Autodesk Inventor part; units mm, degrees
ref_plane "YZ Plane" through (0, 0, 0) normal (1, 0, 0) x (0, 1, 0)
ref_plane "XZ Plane" through (0, 0, 0) normal (0, 1, 0) x (-1, 0, 0)
ref_plane "XY Plane" through (0, 0, 0) normal (0, 0, 1) x (1, 0, 0)
sketch "Sketch1" plane through (0, 0, 0) normal (1, 0, 0) x (0, 1, 0)
  line L0 (1.5875, 103.1875) -> (1.5875, 1.5875)
  line L1 (1.5875, 1.5875) -> (179.3875, 1.5875)
  line L2 (179.3875, 1.5875) -> (179.3875, 7.9375)
  line L3 (179.3875, 7.9375) -> (180.975, 7.9375)
  line L4 (180.975, 7.9375) -> (180.975, 0)
  line L5 (180.975, 0) -> (0, 0)
  line L6 (0, 0) -> (0, 103.1875)
  line L7 (0, 103.1875) -> (1.5875, 103.1875)
  dimension "d0" = 1.5875
  dimension "d1" = 1.5875
  dimension "d2" = 180.975
  dimension "d3" = 101.6
  dimension "d4" = 6.35
extrude "Extrusion1" add sketch "Sketch1" along normal blind 241.3
sketch "Sketch2" plane through (0, 0, 0) normal (0, 0, -1) x (-1, 0, 0)
  line L0 (-241.3, 180.975) -> (-241.3, 0)
  line L1 (0, 0) -> (-241.3, 0)
  line L2 (0, 0) -> (0, 180.975)
  line L3 (-241.3, 127) -> (-215.9, 127)
  line L4 (-215.9, 127) -> (-215.9, 76.2)
  line L5 (-215.9, 76.2) -> (-241.3, 76.2)
  line L6 (-241.3, 76.2) -> (-241.3, 127)
  line L7 (0, 127) -> (-25.4, 127)
  line L8 (-25.4, 127) -> (-25.4, 76.2)
  line L9 (-25.4, 76.2) -> (0, 76.2)
  line L10 (0, 76.2) -> (0, 127)
  dimension "d7" = 25.4
  dimension "d8" = 50.8
  dimension "d9" = 76.2
extrude "Extrusion2" cut sketch "Sketch2" against normal up to next
sketch "Sketch3" plane through (0, 1.5875, 1.5875) normal (0, 0, 1) x (1, 0, 0)
  line L0 (0, 125.4125) -> (25.4, 125.4125)
  line L1 (241.3, 74.6125) -> (215.9, 74.6125)
  line L2 (215.9, 125.4125) -> (214.3125, 125.4125)
  line L3 (214.3125, 125.4125) -> (214.3125, 74.6125)
  line L4 (214.3125, 74.6125) -> (215.9, 74.6125)
  line L5 (215.9, 74.6125) -> (215.9, 125.4125)
  line L6 (25.4, 74.6125) -> (26.9875, 74.6125)
  line L7 (26.9875, 74.6125) -> (26.9875, 125.4125)
  line L8 (26.9875, 125.4125) -> (25.4, 125.4125)
  line L9 (25.4, 125.4125) -> (25.4, 74.6125)
  point P0 (0, -1.5875)
  dimension "d12" = 1.5875
extrude "Extrusion3" add sketch "Sketch3" along normal blind 25.4
sketch "Sketch4" plane through (0, 179.3875, 1.5875) normal (0, 0, 1) x (1, 0, 0)
  line L0 (0, 0) -> (0, -52.3875)
  line L1 (241.3, -177.8) -> (241.3, -103.1875)
  circle A0 centre (228.6, -23.8125) radius 3.1877
  circle A1 centre (228.6, -125.4125) radius 3.1877
  circle A2 centre (12.7, -23.8125) radius 3.1877
  circle A3 centre (12.7, -125.4125) radius 3.1877
  line L2 (12.7, -23.8125) -> (228.6, -23.8125) construction
  line L3 (228.6, -23.8125) -> (228.6, -125.4125) construction
  line L4 (228.6, -125.4125) -> (12.7, -125.4125) construction
  line L5 (12.7, -125.4125) -> (12.7, -23.8125) construction
  line L6 (0, -179.3875) -> (241.3, -179.3875) construction
  line L7 (0, 1.5875) -> (241.3, 1.5875) construction
  dimension "d15" = 6.3754
  dimension "d16" = 12.7
  dimension "d18" = 25.4
  dimension "d19" = 101.6
  dimension "d20" = 12.7
extrude "Extrusion4" cut sketch "Sketch4" against normal through all
sketch "Sketch5" plane through (0, 0, 0) normal (0, -1, 0) x (1, 0, 0)
  line L0 (0, 103.1875) -> (31.75, 103.1875)
  line L1 (31.75, 103.1875) -> (31.75, 71.4375)
  line L2 (31.75, 71.4375) -> (0, 71.4375)
  line L3 (0, 71.4375) -> (0, 103.1875)
  line L4 (241.3, 103.1875) -> (209.55, 103.1875)
  line L5 (209.55, 103.1875) -> (209.55, 71.4375)
  line L6 (209.55, 71.4375) -> (241.3, 71.4375)
  line L7 (241.3, 71.4375) -> (241.3, 103.1875)
  dimension "d23" = 31.75
extrude "Extrusion5" cut sketch "Sketch5" against normal up to next
sketch "Sketch6" plane through (0, 1.5875, 1.5875) normal (0, 1, 0) x (1, 0, 0)
  line L0 (209.55, -101.6) -> (209.55, -69.85)
  line L1 (31.75, -69.85) -> (31.75, -101.6)
  line L2 (31.75, -101.6) -> (209.55, -101.6)
  circle A0 centre (76.2, -88.9) radius 3.175
  circle A1 centre (165.1, -88.9) radius 3.175
  line L3 (165.1, -88.9) -> (209.55, -88.9) construction
  line L4 (76.2, -88.9) -> (31.75, -88.9) construction
  point P0 (0, 1.5875)
  dimension "d26" = 12.7
  dimension "d27" = 12.7
  dimension "d28" = 88.9
  dimension "d29" = 6.35
extrude "Extrusion6" cut sketch "Sketch6" against normal up to next
properties part number "BatteryMount" material "Aluminum-6061"
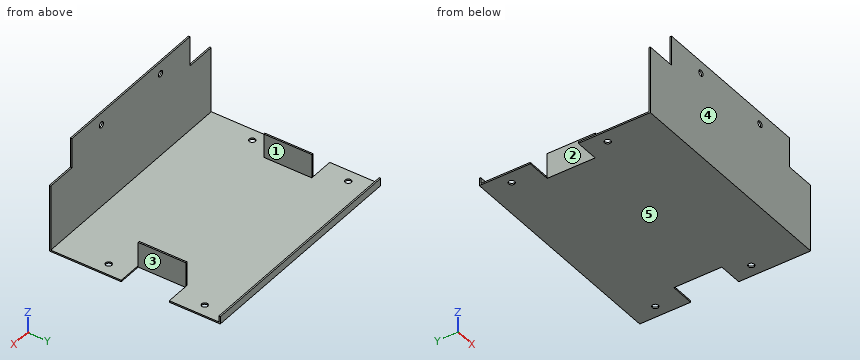
Geometry: final body of the model. Coordinates: model frame, mm. Face numbers are marked on the shaded views. A direction names the side the tool comes from. Round coordinates to 2 decimals unless told otherwise and drop trailing zeros. Order: outer loops, then holes, each group sorted by start corner. A loop starts at its lowest first (then second) coordinate and runs counter-clockwise, first axis right, second up. Notation, with made-up numbers: (-24, -20) -> (3, -20) arc R27 ccw to (3, 5) -> close; hole circle Ø4 at (-40, 10.25). An arc over 180 degrees is marked (long way). Use one line per item in the form item = value.
(1) Draft query along Y for the marked faces 3, 4 and 5. Return one class per face: pulls with the +Y half, pulls with the -Y half, needs draft (parallel to the pull), parting line crosses it, or undercut.
Results list:
face_3 = undercut
face_4 = pulls with the -Y half
face_5 = needs draft
(2) Section C-C on y = 94.5. Return loops of the section in (x, z), and give its area (3 significant figures).
Results list:
outline = (25.4, 0) -> (215.9, 0) -> (215.9, 26.99) -> (214.31, 26.99) -> (214.31, 1.59) -> (26.99, 1.59) -> (26.99, 26.99) -> (25.4, 26.99) -> close
area = 383 mm^2
(3) Ray query, probe 1 along Y at (x, z) = (228.6, 0.8) (3 decimals); probe 2 along Z at (x, y) = (165.1, 0.95); probe 3 along Y at (x, z) = (117.5, 5.5) (1 decimal). Return the intervals inside material, ascending. Write a range as [from, to].
Results list:
probe_1 = [0, 50.787], [57.163, 76.2], [127, 152.387], [158.763, 180.975]
probe_2 = [0, 87.31], [93.66, 103.19]
probe_3 = [0, 1.6], [179.4, 181]
(4) Section B-B on x = 76.2. Return loops of the section in (y, z) (1 decimal), and give its area (3 significant figures).
Results list:
outline = (0, 0) -> (181, 0) -> (181, 7.9) -> (179.4, 7.9) -> (179.4, 1.6) -> (1.6, 1.6) -> (1.6, 87.3) -> (0, 87.3) -> close; (0, 93.7) -> (1.6, 93.7) -> (1.6, 103.2) -> (0, 103.2) -> close
area = 449 mm^2
(5) Section D-D on x = 36.5. Return loops of the section in (y, z) (1 decimal), and give its area (3 significant figures).
Results list:
outline = (0, 0) -> (181, 0) -> (181, 7.9) -> (179.4, 7.9) -> (179.4, 1.6) -> (1.6, 1.6) -> (1.6, 103.2) -> (0, 103.2) -> close
area = 459 mm^2
(6) Section A-A on x = 228.6. Return loops of the section in (y, z) (1 decimal).
Results list:
outline = (0, 0) -> (50.8, 0) -> (50.8, 1.6) -> (1.6, 1.6) -> (1.6, 71.4) -> (0, 71.4) -> close; (57.2, 0) -> (76.2, 0) -> (76.2, 1.6) -> (57.2, 1.6) -> close; (127, 0) -> (152.4, 0) -> (152.4, 1.6) -> (127, 1.6) -> close; (158.8, 0) -> (181, 0) -> (181, 7.9) -> (179.4, 7.9) -> (179.4, 1.6) -> (158.8, 1.6) -> close
(7) First-contact query: pin 1 Ø8 at (x, z) = (82, 63) entering from +Y; pin 2 Ø1.3 at (x, y) = (22.5, 1) entering from +Z; pin 3 Ø5 at (x, y) = (228.6, 53.975) entering from -Z; pin 4 Ø1.3 at (x, z) = (215, 11) entering from +Y. Flat tips, straight axial feed; report the tip coordinate or a pass-through.
Results list:
pin_1 = 1.59
pin_2 = 71.44
pin_3 = through
pin_4 = 127
(8) Access query for the marked faces 1 and 2. Directions: +Z, -Z, +X, -X, +Y, -Y. A direction counts if a zero-diameter tool reaches every point of the face in a straight line with its end or side. Return the directions, or none.
Results list:
face_1 = +Z
face_2 = +Z, -Z, -X
